```python
from build123d import *

# Parameters (mm, degrees)
BOSS_EXTRUDE1_DEPTH = 3
BOSS_EXTRUDE2_DEPTH = 3


with BuildPart() as part:
    # Sketch1 → Boss-Extrude1 (new body)
    with BuildSketch(Plane(origin=(0, 0, 0), x_dir=(0, 0, -1), z_dir=(1, 0, 0))):
        with BuildLine():
            Line((-7.997844187, 2.375), (-7.997844187, -2))
            Line((-7.997844187, -2), (7.997844187, -2))
            Line((7.997844187, -2), (7.997844187, 2.375))
            ThreePointArc((7.997844187, 2.375), (3.423879317, 6.186439769), (0.5, 1))
            Line((0.5, 1), (2.186352513, 1))
            ThreePointArc((2.186352513, 1), (3.401228889, 4.637718799), (6.497844187, 2.375))
            Line((6.497844187, 2.375), (6.497844187, 0))
            Line((6.497844187, 0), (-6.497844187, 0))
            Line((-6.497844187, 0), (-6.497844187, 2.375))
            ThreePointArc((-6.497844187, 2.375), (-3.401228889, 4.637718799), (-2.186352513, 1))
            Line((-2.186352513, 1), (-0.5, 1))
            ThreePointArc((-0.5, 1), (-3.423879317, 6.186439769), (-7.997844187, 2.375))
        make_face()
    extrude(amount=BOSS_EXTRUDE1_DEPTH)

    # Sketch2 → Boss-Extrude2 (add)
    with BuildSketch(Plane.ZY):
        Polygon((-7.997844187, -2), (-7.997844187, -7.1), (0, -7.1), (0, -5.1), (-4.997844187, -5.1), (-4.997844187, -2), align=None)
    extrude(amount=-BOSS_EXTRUDE2_DEPTH)


solid = part.part
```
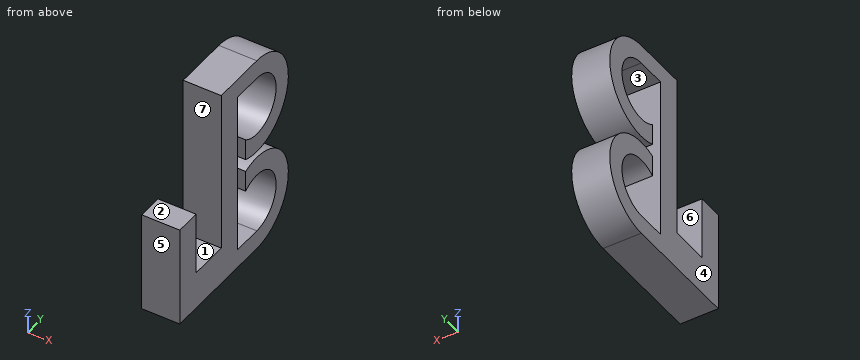
For this review, take the finished solid that the model builds, in its own axes (mm). Face numbers are marked on the shaded views. A direction names the side the tool comes from. Coordinates: 2 decimals unless noted, no trailing zeros. Loops run counter-clockwise (first coordinate to the right, second up) from the corner with the lowest first, then second, coordinate; pieces in that order, holes last.
1. Add section B-B, the plane z = 1.25. Give the boundary of the cut face in (x, y).
2. Add section C-C, the plane y = 5. Give the boundary of the cut face in (x, z).
3. Mouldability with a two-part tool opening along Y and no side actions: class the marked faces 4, 5, 6 and 7 as +Y half, -Y half, draft (parallel to the pull), parting line (faces both ways), or undercut.
4. For the marked faces 1, 2 and 3, list the 3-axis set-ups (+Z, -Z, +X, -X, +Y, -Y) from which the entire face can be reached by the end or side of a thin tool; tool diameter is ignored.
5. Add section D-D, the plane z = -0.75. Give the boundary of the cut face in (x, y), then the cut area to 3 significant figures.
6. Insertion check: P1, Ø4, axis at y = 2.37, z = 4.12, coming from the -X side; P2, Ø1.5, axis at x = 1, z = -2.5, coming from the +Y side; P3, Ø0.8, axis at x = 2, z = 1, coming from the -Y side; P4, Ø0.9, axis at x = 1.5, y = -4, coming from the +Z side. Each pin has a flat end and moves straight along its axis. Give the tip position at first contact, or say it passes through.
7. Add section A-A, the plane y = 3.25. Give the boundary of the cut face in (x, z), then the cut area to 3 significant figures.
8. For line 1 (Z direction, x = 0.8, y = 0.5); line 2 (Y direction, x = 1.1, z = -2.75); line 3 (Z direction, x = 1.25, y = 1.25), list the stretches that pass through material, from the lowest coordinate up.
Result:
1. outline: (0, -2) - (3, -2) - (3, 0) - (0, 0) - close; (0, 1) - (3, 1) - (3, 4.98) - (0, 4.98) - close
2. outline: (0, -6.97) - (3, -6.97) - (3, -1.27) - (0, -1.27) - close; (0, 1.27) - (3, 1.27) - (3, 6.97) - (0, 6.97) - close
3. face 4: draft
3. face 5: -Y half
3. face 6: undercut
3. face 7: undercut
4. face 1: +Z, +X, -X
4. face 2: +Z, +X, -X, -Y
4. face 3: +X, -X
5. outline: (0, -7.1) - (3, -7.1) - (3, -5.1) - (0, -5.1) - close; (0, -2) - (3, -2) - (3, 0) - (0, 0) - close; (0, 1) - (3, 1) - (3, 4.28) - (0, 4.28) - close
5. area: 21.8 mm2
6. P1: passes through
6. P2: stops at y = 6.15
6. P3: stops at y = -2
6. P4: stops at z = -5
7. outline: (0, -7.9) - (3, -7.9) - (3, -6.33) - (0, -6.33) - close; (0, -1.91) - (3, -1.91) - (3, -0.35) - (0, -0.35) - close; (0, 0.35) - (3, 0.35) - (3, 1.91) - (0, 1.91) - close; (0, 6.33) - (3, 6.33) - (3, 7.9) - (0, 7.9) - close
7. area: 18.8 mm2
8. line 1: z = -8 to -6.5, 6.5 to 8
8. line 2: y = -7.1 to -5.1, -2 to 0, 4.31 to 6
8. line 3: z = -8 to -6.5, -2.03 to -0.41, 0.41 to 2.03, 6.5 to 8
